Answer from the drawing. Dimensions are ordinates in mm from the lowest x, y and z of the part. A direction names the side the tool comes from. Round coordinates to 2 decimals unless told otherwise and drop trailing zeros. Order: outer loops, then holes, each group sorted by start corner. A loop starts at its lowest first (then second) coordinate and runs counter-clockwise, first axis right, second up.
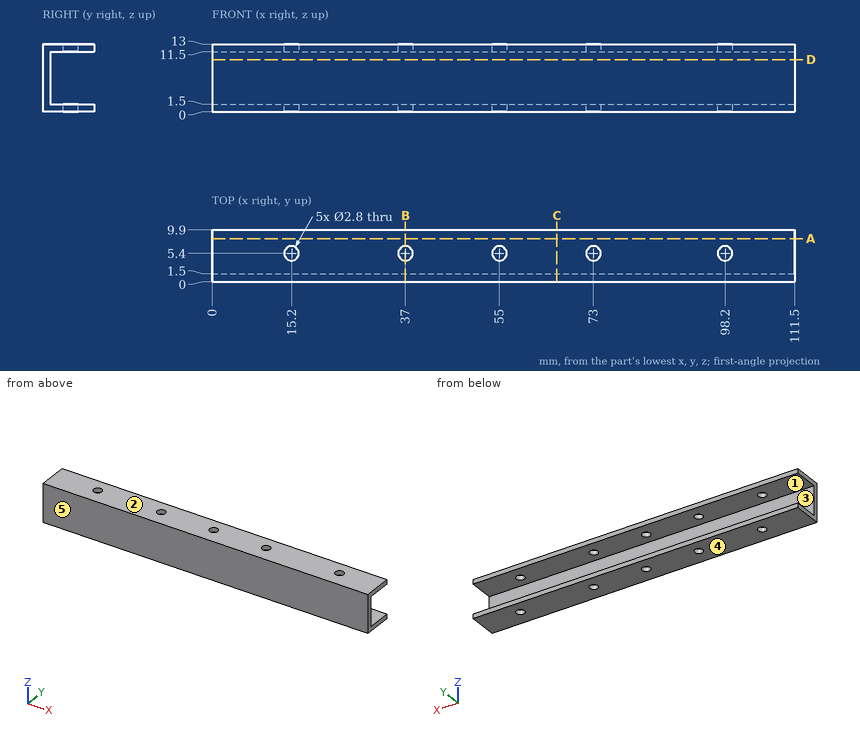
Q1. For a pull along Z with two mould halves and no side action, classify the marked faces 3, 4 and 5 as released by +Z, released by -Z, zero draft, split by the parting line, or undercut.
Outcome:
face 3: undercut
face 4: released by -Z
face 5: zero draft
Q2. Straight lines are drawn through the part: probe 1 along X at (y, z) = (5.5, 1); probe 2 along Z at (x, y) = (46, 2.25); probe 3 along Y at (x, z) = (55, 11.9). For each, find the intervals that lie inside material, in ascending order.
Outcome:
probe 1: x = 0 to 13.8, 16.6 to 35.6, 38.4 to 53.6, 56.4 to 71.6, 74.4 to 96.8, 99.6 to 111.5
probe 2: z = 0 to 1.5, 11.5 to 13
probe 3: y = 0 to 4, 6.8 to 9.9
Q3. For the marked faces 1 and 2, determine the directions among +Z, -Z, +X, -X, +Y, -Y from which every point of the face is accessible in a straight line to the end or side of a thin tool.
Outcome:
face 1: +X, -X, +Y
face 2: +Z, +X, -X, +Y, -Y
Q4. A cutting plane is placed at C-C, the plane x = 66. Give the vertices of the cut face in (y, z).
Outcome:
outline: (0, 0) - (9.9, 0) - (9.9, 1.5) - (1.5, 1.5) - (1.5, 11.5) - (9.9, 11.5) - (9.9, 13) - (0, 13) - close
Q5. A cutting plane is placed at D-D, the plane z = 10. Give the vertices of the cut face in (x, y).
Outcome:
outline: (0, 0) - (111.5, 0) - (111.5, 1.5) - (0, 1.5) - close
Q6. A cutting plane is placed at A-A, the plane y = 8.25. Give the vertices of the cut face in (x, z).
Outcome:
outline: (0, 0) - (111.5, 0) - (111.5, 1.5) - (0, 1.5) - close; (0, 11.5) - (111.5, 11.5) - (111.5, 13) - (0, 13) - close
Q7. A cutting plane is placed at B-B, the plane x = 37. Give the vertices of the cut face in (y, z), plus the area to 3 significant figures.
Outcome:
outline: (0, 0) - (4, 0) - (4, 1.5) - (1.5, 1.5) - (1.5, 11.5) - (4, 11.5) - (4, 13) - (0, 13) - close; (6.8, 0) - (9.9, 0) - (9.9, 1.5) - (6.8, 1.5) - close; (6.8, 11.5) - (9.9, 11.5) - (9.9, 13) - (6.8, 13) - close
area: 36.3 mm2
Q8. Flat-ended cylindrical pins translate along their axes: pin 1 (3.5 mm diameter, centred on x = 55, y = 5.4, fed in from +Z); pin 2 (3 mm diameter, centred on x = 39.5, z = 8.5, fed in from +Y). Find the tip coordinate at first contact, or state that the pin passes through.
Outcome:
pin 1: stops at z = 13
pin 2: stops at y = 1.5
